Build history of the part. All positions in model axes, mm. Face numbers are marked on the shaded views. A direction names the side the tool comes from. Give positions to 0.01 mm unless a question says otherwise; leave off trailing zeros. Order: outer loops, then holes, each group sorted by start corner. A loop starts at its lowest first (then second) coordinate and runs counter-clockwise, first axis right, second up. Notation, with made-up numbers: (38, -25) - (71, -25) arc R27 cw to (71, -8) - close; hole circle Ø6 at (42.25, -21.75). An arc over 180 degrees is marked (long way). Write each question's results on one line, items separated by ' | '. Start each with the question number.
1) Cut at A-A on z = 9. List the corners of the cut face in (x, y).
2) Tool access for the marked faces 5, 6, 7 and 8: list every direction of +Z, -Z, +X, -X, +Y, -Y with a clear straight run to the whole face (end or side of a thin tool).
3) Cut at B-B on x = 7.25. List the corners of the cut face in (y, z).
4) Two-plate mould, pull along X, no slides. Class the marked faces 1, 2, 3 and 4: +X half, -X half, draft (parallel to the pull), parting line (faces both ways), or undercut.
5) Drop flat-ended pins along their axis: pin 1 Ø5.5 at (x, y) = (-2, -2) entering from +Z; pin 2 Ø0.9 at (x, z) = (-1.5, 10) entering from -Y; pin 3 Ø1 at (y, z) = (-4, 7) entering from -X. Give the stop position or say it passes through.
6) Drill centre lines: line 1 along Z through (x, y) = (8.75, -1.75); line 2 along Y through (x, z) = (1.5, 11.5); line 3 along Y through (x, z) = (4, 6.5). Where is each one in solid material? Low to high. Write a range as from..to.
7) Cut at C-C on z = 5.5. State how many separate pieces and enclosed holes the cut face has, plus the area to 3 significant figures.
from build123d import *

# Parameters (mm, degrees)
F0_W      = 20
F0_H      = 20
F1_DEPTH  = 3
F2_W      = 0.2
F2_H      = 5
F3_DEPTH  = 10
F4_DEPTH  = 0.1
F5_DEPTH  = 0.4
F6_DEPTH  = 0.5
F7_DEPTH  = 0.6
F8_DEPTH  = 0.7
F9_DEPTH  = 4
F10_W     = 0.2
F10_H     = 5
F10_W_2   = 0.4
F10_W_3   = 0.8
F10_W_4   = 1
F10_W_5   = 1.2
F10_W_6   = 1.4
F11_DEPTH = 7
F12_R     = 0.8


with BuildPart() as f1:
    # F0 (on Top) → F1 (new body)
    with BuildSketch(Plane.XY):
        Rectangle(F0_W, F0_H)
    extrude(amount=F1_DEPTH)

    # F2 (on face) → F3 (join)
    with BuildSketch(Plane.XY.offset(3)):
        with Locations((-7.4, 5)):
            Rectangle(F2_W, F2_H)
        with Locations((-4.44, 5)):
            Rectangle(F2_W, F2_H)
        with Locations((-1.48, 5)):
            Rectangle(F2_W, F2_H)
        with Locations((1.48, 5)):
            Rectangle(F2_W, F2_H)
        with Locations((4.44, 5)):
            Rectangle(F2_W, F2_H)
        with Locations((7.4, 5)):
            Rectangle(F2_W, F2_H)
    extrude(amount=F3_DEPTH)

    # F4 (add, symmetric): faces of the model
    f4_faces = [f1.faces().sort_by_distance(p)[0] for p in [
        (-4.54, 5, 8),
        (-4.34, 5, 8),
    ]]
    extrude(f4_faces, amount=F4_DEPTH, both=True, dir=(-1, 0, 0))

    # F5 (add, symmetric): a face of the model
    f5_faces = [f1.faces().sort_by_distance(p)[0] for p in [
        (-1.58, 5, 8),
    ]]
    extrude(f5_faces, amount=F5_DEPTH, both=True)

    # F6 (add, symmetric): a face of the model
    f6_faces = [f1.faces().sort_by_distance(p)[0] for p in [
        (1.38, 5, 8),
    ]]
    extrude(f6_faces, amount=F6_DEPTH, both=True)

    # F7 (add, symmetric): a face of the model
    f7_faces = [f1.faces().sort_by_distance(p)[0] for p in [
        (4.34, 5, 8),
    ]]
    extrude(f7_faces, amount=F7_DEPTH, both=True)

    # F8 (add, symmetric): a face of the model
    f8_faces = [f1.faces().sort_by_distance(p)[0] for p in [
        (7.3, 5, 8),
    ]]
    extrude(f8_faces, amount=F8_DEPTH, both=True)

    # F9 (add): a face of the model
    f9_faces = [f1.faces().sort_by_distance(p)[0] for p in [
        (-0.16384, -0.3333333333, 3),
    ]]
    extrude(f9_faces, amount=F9_DEPTH)

    # F10 (on face) → F11 (cut, through all)
    with BuildSketch(Plane.XY.offset(7)):
        with Locations((-7.4, -5)):
            Rectangle(F10_W, F10_H)
        with Locations((-4.44, -5)):
            Rectangle(F10_W_2, F10_H)
        with Locations((-1.58, -5)):
            Rectangle(F10_W_3, F10_H)
        with Locations((1.38, -5)):
            Rectangle(F10_W_4, F10_H)
        with Locations((4.34, -5)):
            Rectangle(F10_W_5, F10_H)
        with Locations((7.3, -5)):
            Rectangle(F10_W_6, F10_H)
    extrude(amount=-F11_DEPTH, mode=Mode.SUBTRACT)

    # F12
    f12_edges = [f1.edges().sort_by_distance(p)[0] for p in [
        (10, -10, 3.5),
        (-10, -10, 3.5),
        (-10, 10, 3.5),
        (10, 10, 3.5),
        (-10, 0, 7),
        (0, 10, 7),
        (0, -10, 7),
        (10, 0, 7),
        (-7.5, 5, 7),
        (-7.3, 5, 7),
        (-4.64, 5, 7),
        (-4.24, 5, 7),
        (-1.98, 5, 7),
        (-1.18, 5, 7),
        (0.88, 5, 7),
        (1.88, 5, 7),
        (3.74, 5, 7),
        (6.6, 5, 7),
        (4.94, 5, 7),
        (8, 5, 7),
        (-7.4, 7.5, 7),
        (-7.4, 2.5, 7),
        (-4.44, 2.5, 7),
        (-1.58, 2.5, 7),
        (1.38, 2.5, 7),
        (4.34, 2.5, 7),
        (7.3, 2.5, 7),
        (7.3, -2.5, 7),
        (8, -5, 7),
        (6.6, -5, 7),
        (7.3, -7.5, 7),
        (4.94, -5, 7),
        (4.34, -2.5, 7),
        (4.34, -7.5, 7),
        (3.74, -5, 7),
        (1.88, -5, 7),
        (1.38, -2.5, 7),
        (1.38, -7.5, 7),
        (0.88, -5, 7),
        (-1.18, -5, 7),
        (-1.98, -5, 7),
        (-1.58, -2.5, 7),
        (-1.58, -7.5, 7),
        (-4.24, -5, 7),
        (-4.44, -2.5, 7),
        (-4.64, -5, 7),
        (-4.44, -7.5, 7),
        (-7.3, -5, 7),
        (-7.5, -5, 7),
        (-7.4, -2.5, 7),
        (-7.4, -7.5, 7),
        (-4.44, 7.5, 7),
        (-1.58, 7.5, 7),
        (1.38, 7.5, 7),
        (4.34, 7.5, 7),
        (7.3, 7.5, 7),
    ]]
    fillet(f12_edges, radius=F12_R)


solid = f1.part
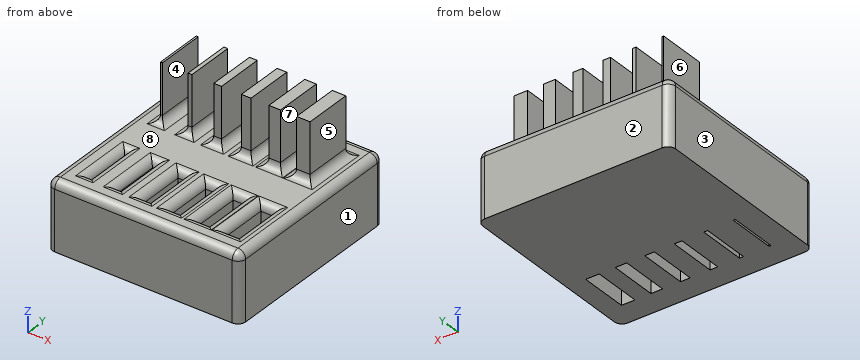
Results:
1) outline: (-7.5, 2.5) - (-7.3, 2.5) - (-7.3, 7.5) - (-7.5, 7.5) - close; (-4.64, 2.5) - (-4.24, 2.5) - (-4.24, 7.5) - (-4.64, 7.5) - close; (-1.98, 2.5) - (-1.18, 2.5) - (-1.18, 7.5) - (-1.98, 7.5) - close; (0.88, 2.5) - (1.88, 2.5) - (1.88, 7.5) - (0.88, 7.5) - close; (3.74, 2.5) - (4.94, 2.5) - (4.94, 7.5) - (3.74, 7.5) - close; (6.6, 2.5) - (8, 2.5) - (8, 7.5) - (6.6, 7.5) - close
2) face 5: +Z, +X, +Y, -Y | face 6: +Z, -X, +Y, -Y | face 7: +Z, +Y, -Y | face 8: +Z
3) outline: (-10, 0) - (-7.5, 0) - (-7.5, 6.2) arc R0.8 ccw to (-8.3, 7) - (-9.2, 7) arc R0.8 ccw to (-10, 6.2) - close; (-2.5, 0) - (10, 0) - (10, 6.2) arc R0.8 ccw to (9.2, 7) - (8.3, 7) arc R0.8 cw to (7.5, 7.8) - (7.5, 13) - (2.5, 13) - (2.5, 7.8) arc R0.8 cw to (1.7, 7) - (-1.7, 7) arc R0.8 ccw to (-2.5, 6.2) - close
4) face 1: +X half | face 2: draft | face 3: -X half | face 4: undercut
5) pin 1: z = 7 | pin 2: y = 2.5 | pin 3: x = -9.94
6) line 1: 0..7 | line 2: 2.5..7.5 | line 3: -9.94..-7.56, -2.44..9.94
7) separate pieces: 1 | enclosed holes: 6 | area: 374 mm^2
